Work out the finished part from the listing and answer in its coordinate system (mm). Round coordinates to 2 decimals unless told otherwise and drop trailing zeros. Loops run counter-clockwise (first coordinate to the right, second up) from the corner with the lowest first, then second, coordinate; pieces in that order, holes last.
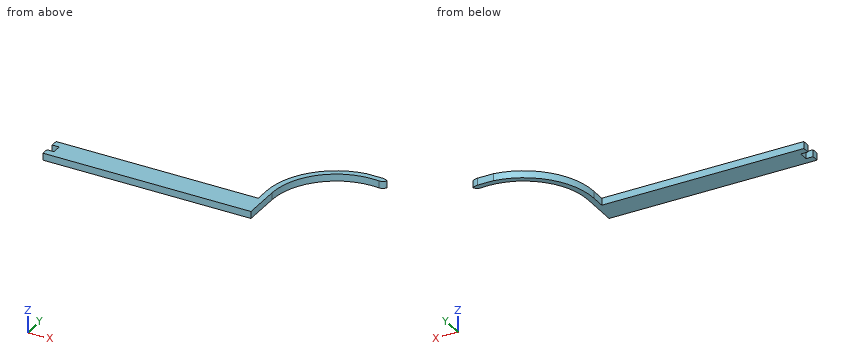
```python
from build123d import *

# Parameters (mm, degrees)
EXTRUDE_1_DEPTH = 6


with BuildPart() as part:
    # Эскиз2 → Бобышка-Вытянуть1 (new body)
    with BuildSketch(Plane.XY):
        with BuildLine():
            Line((0, 20), (167, 20))
            Line((167, 20), (167, 32))
            ThreePointArc((167, 32), (182.048214587, 71.740873017), (219.644566271, 91.547439867))
            Line((219.644566271, 91.547439867), (233, 91.547439867))
            ThreePointArc((233, 91.547439867), (235.649529771, 91.095949123), (238, 89.792437865))
            ThreePointArc((238, 89.792437865), (235.982168822, 87.370794766), (232.906213145, 86.681959057))
            ThreePointArc((232.906213145, 86.681959057), (190.256576935, 72.925797017), (172, 32))
            Line((172, 32), (172, 0))
            Line((172, 0), (0, 0))
            Line((0, 0), (-6, 0))
            Line((-6, 0), (-6, 6))
            Line((-6, 6), (0, 6))
            Line((0, 6), (0, 14))
            Line((0, 14), (-6, 14))
            Line((-6, 14), (-6, 20))
            Line((-6, 20), (0, 20))
        make_face()
    extrude(amount=EXTRUDE_1_DEPTH)


solid = part.part
```
1. Given pin 1 (3 mm diameter, centred on x = 111.5, z = 3.5, fed in from +Y); pin 2 (1.8 mm diameter, centred on y = 9, z = 4.5, fed in from -X); pin 3 (10 mm diameter, centred on x = 157.5, y = 37.5, fed in from -Z); pin 4 (2 mm diameter, centred on y = 72, z = 1, fed in from -X), each flat-ended and moving along its own axis, determine where each tip first touches the part or whether it passes through.
Answer key:
pin 1: stops at y = 20
pin 2: stops at x = 0
pin 3: passes through
pin 4: stops at x = 181.4
2. Find section A-A (x = 93.5). Write down the section's boundary in (y, z), then the cut area to 3 significant figures.
Answer key:
outline: (0, 0) - (20, 0) - (20, 6) - (0, 6) - close
area: 120 mm2
3. Find section B-B (z = 3.8). Write down the section's boundary in (x, y).
Answer key:
outline: (-6, 0) - (172, 0) - (172, 32) arc R55 cw to (232.91, 86.68) arc R4.89 ccw to (238, 89.79) arc R8 ccw to (233, 91.55) - (219.64, 91.55) arc R60 ccw to (167, 32) - (167, 20) - (-6, 20) - (-6, 14) - (0, 14) - (0, 6) - (-6, 6) - close
4. Find section C-C (y = 80). Write down the section's boundary in (x, z).
Answer key:
outline: (191, 0) - (200.15, 0) - (200.15, 6) - (191, 6) - close
5. Consider probe 1 along Y at (x, z) = (56, 1.1); probe 2 along X at (y, z) = (11.5, 2.35); probe 3 along X at (y, z) = (23, 4.55). Determine where each line is inside the solid, lowest interval first.
Answer key:
probe 1: y = 0 to 20
probe 2: x = 0 to 172
probe 3: x = 167 to 172
